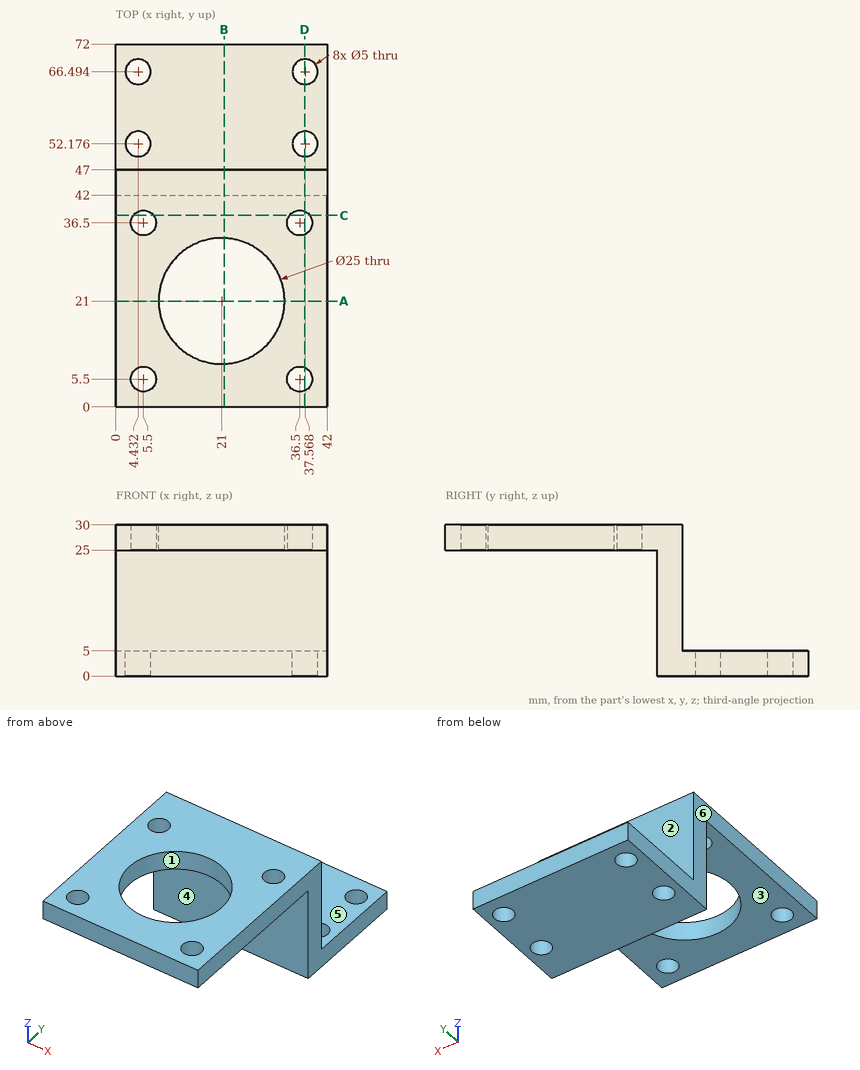
Source: three-view drawing plus pictorial views. Frame: mm from the lowest corner of the part. A direction names the side the tool comes from. Give positions to 0.01 mm unless a question says otherwise; leave off trailing zeros. Loops run counter-clockwise (first coordinate to the right, second up) from the corner with the lowest first, then second, coordinate; pieces in that order, holes last. Notation, with made-up numbers: (-38, -25) -> (-15, -25) arc R13 cw to (-15, -16) -> close; hole circle Ø2 at (1, 53.25). An arc over 180 degrees is marked (long way). Use a Markdown table: item, result. Add a question column.
(1) Section query C-C (y = 38). Output: boundary loops of the cut face in (x, z).
(2) Access query for the marked faces 4, 5 and 6. Directions: +Z, -Z, +X, -X, +Y, -Y. A direction counts if a zero-diameter tool reaches every point of the face in a straight line with its end or side. Return the directions, or none.
(3) Section query A-A (y = 21). Output: boundary loops of the cut face in (x, z).
(4) Ray query, line 1 (Y direction, x = 36.5, z = 27.55); line 2 (X direction, y = 52, z = 2.25) (1 decimal); line 3 (Y direction, x = 21, z = 28.8). Return the intervals inside material, ascending.
(5) Section query D-D (x = 37.5). Output: boundary loops of the cut face in (y, z) (1 decimal), then the cut area to 3 significant figures.
(6) Section query B-B (x = 21.5). Output: boundary loops of the cut face in (y, z).
(7) Pull-direction query (Y, two-part tool) for the marked faces 1, 2 and 3; classes: +Y half, -Y half, draft (parallel to the pull), parting line (faces both ways), or undercut.
(8) First-contact query: pin 1 Ø7.5 at (x, z) = (14.5, 13.5) entering from +Y; pin 2 Ø8 at (x, y) = (18.5, 33.5) entering from -Z; pin 3 Ø20 at (x, y) = (18, 57.5) entering from +Z. Flat tips, straight axial feed; report the tip coordinate or a pass-through.
Checked values:
| question | item | result |
|---|---|---|
| 1 | outline | (0, 25) -> (3.5, 25) -> (3.5, 30) -> (0, 30) -> close; (7.5, 25) -> (34.5, 25) -> (34.5, 30) -> (7.5, 30) -> close; (38.5, 25) -> (42, 25) -> (42, 30) -> (38.5, 30) -> close |
| 2 | face 4 | -Z, +X, -X, -Y |
| 2 | face 5 | +Z, +X, -X, +Y |
| 2 | face 6 | +Z, -Z, -X, +Y, -Y |
| 3 | outline | (0, 25) -> (8.5, 25) -> (8.5, 30) -> (0, 30) -> close; (33.5, 25) -> (42, 25) -> (42, 30) -> (33.5, 30) -> close |
| 4 | line 1 | 0 to 3, 8 to 34, 39 to 47 |
| 4 | line 2 | 0 to 1.9, 6.9 to 35.1, 40.1 to 42 |
| 4 | line 3 | 0 to 8.5, 33.5 to 47 |
| 5 | outline | (0, 25) -> (3.2, 25) -> (3.2, 30) -> (0, 30) -> close; (7.8, 25) -> (34.2, 25) -> (34.2, 30) -> (7.8, 30) -> close; (38.8, 25) -> (42, 25) -> (42, 0) -> (49.7, 0) -> (49.7, 5) -> (47, 5) -> (47, 30) -> (38.8, 30) -> close; (54.7, 0) -> (64, 0) -> (64, 5) -> (54.7, 5) -> close; (69, 0) -> (72, 0) -> (72, 5) -> (69, 5) -> close |
| 5 | area | 389 mm^2 |
| 6 | outline | (0, 25) -> (8.51, 25) -> (8.51, 30) -> (0, 30) -> close; (33.49, 25) -> (42, 25) -> (42, 0) -> (72, 0) -> (72, 5) -> (47, 5) -> (47, 30) -> (33.49, 30) -> close |
| 7 | face 1 | undercut |
| 7 | face 2 | +Y half |
| 7 | face 3 | draft |
| 8 | pin 1 | y = 47 |
| 8 | pin 2 | z = 25 |
| 8 | pin 3 | z = 5 |
